For this review, take the finished solid that the model builds, in its own axes (mm). A direction names the side the tool comes from. Give positions to 0.01 mm unless a question says otherwise; leave off trailing zeros. Loops run counter-clockwise (first coordinate to the right, second up) from the corner with the lowest first, then second, coordinate; pieces in that order, holes last.
Autodesk Inventor part; units mm, degrees
ref_plane "Work Plane1" through (-110.3759, -8.6414, 0) normal (0, 1, 0) x (1, 0, 0)
ref_plane "YZ Plane" through (0, 0, 0) normal (1, 0, 0) x (0, 1, 0)
ref_plane "XZ Plane" through (0, 0, 0) normal (0, 1, 0) x (-1, 0, 0)
sketch "Sketch1" plane through (0, 0, 0) normal (0, 0, 1) x (1, 0, 0)
  line L0 (-110.3759, -8.6414) -> (42.0241, -8.6414)
  line L1 (42.0241, -8.6414) -> (42.0241, -59.4414)
  line L2 (42.0241, -59.4414) -> (-110.3759, -59.4414)
  circle A0 centre (-46.8759, -24.5164) radius 3.2512
  circle A1 centre (-46.8759, -43.5664) radius 3.2512
  line L3 (-13.5384, -25.7986) -> (-4.0134, -25.7986)
  line L4 (-4.0134, -25.7986) -> (0.7491, -34.0475)
  line L5 (0.7491, -34.0475) -> (-4.0134, -42.2964)
  line L6 (-4.0134, -42.2964) -> (-13.5384, -42.2964)
  line L7 (-13.5384, -42.2964) -> (-18.3009, -34.0475)
  line L8 (-18.3009, -34.0475) -> (-13.5384, -25.7986)
  circle A2 centre (-110.3759, -34.0414) radius 3.9751
  arc A3 (-110.3759, -8.6414) -> (-110.3759, -59.4414) centre (-110.3759, -34.0414) ccw
  point P0 (0, 0)
  point P1 (-8.7759, -34.0414)
  point P2 (-8.7759, -42.2964)
  dimension "d4" = 6.5024
  dimension "d5" = 6.5024
  dimension "d9" = 152.4
  dimension "d10" = 9.525
  dimension "d11" = 9.525
  dimension "d13" = 120
  dimension "d16" = 9.525
  dimension "d17" = 9.525
  dimension "d18" = 120
  dimension "d19" = 9.525
  dimension "d20" = 9.525
  dimension "d21" = 50.8
  dimension "d22" = 8.255
  dimension "d23" = 9.525
  dimension "d25" = 7.9502
  dimension "d27" = 9.525
  dimension "d37" = 19.05
  dimension "d38" = 50.8
  dimension "d39" = 25.4
  dimension "d40" = 63.5
  dimension "d51" = 101.6
extrude "Extrusion1" add sketch "Sketch1" along normal blind 10.16
ref_plane "Work Plane1" through (-110.3759, -8.6414, 0) normal (0, 1, 0) x (1, 0, 0)
sketch "Sketch3" plane through (-110.3759, -8.6414, 0) normal (0, 1, 0) x (1, 0, 0)
  line L0 (50.8, 1.8056) -> (50.8, -17.2484)
  line L1 (152.4, 0) -> (152.4, -10.16)
  circle A0 centre (76.2, -5.08) radius 3.175
  point P0 (110.3759, 0)
  point P1 (152.4, -5.08)
  dimension "d46" = 101.6
  dimension "d47" = 6.35
  dimension "d48" = 25.4
extrude "Extrusion2" cut sketch "Sketch3" against normal blind 50.8
sketch "Sketch4" plane through (42.0241, -59.4414, 0) normal (1, 0, 0) x (0, 0, -1)
  line L0 (-10.16, 0) -> (-10.16, 50.8)
  line L1 (0, 0) -> (0, 50.8)
  line L2 (-10.16, 50.8) -> (0, 50.8)
  line L3 (0, 50.8) -> (0, 0)
  line L4 (0, 0) -> (-10.16, 0)
  line L5 (-10.16, 0) -> (-10.16, 50.8)
  point P0 (0, 59.4414)
  point P1 (-10.16, 0)
extrude "Extrusion3" cut sketch "Sketch4" against normal blind 38.1
properties part number "new plates for arm"
Item 1: Tool access review of faces 1 (the flat face through (-54, -8.641, 5)), 2 (the flat face through (-1.665, -29.865, 5.009)): name each direction out of +Z, -Z, +X, -X, +Y, -Y from which nothing blocks a thin tool from reaching the whole face with its end or side.
Answer:
face 1: +Z, -Z, +X, -X, +Y
face 2: +Z, -Z
Item 2: Take a section at C-C on y = -19. Give the boundary of the cut face in (x, z) (3 decimals), and give its area (3 significant figures).
Answer:
outline: (-130.843, 0) - (3.924, 0) - (3.924, 10.16) - (-130.843, 10.16) - close; hole circle Ø6.35 at (-34.176, 5.08)
area: 1,340 mm2
Item 3: For L1, parallel to Y at x = -9, z = 7.25; L2, parallel to X at y = -42, z = 6.5; L3, parallel to X at y = -31, z = 5.08, list the stretches that pass through material, from the lowest coordinate up.
Answer:
L1: y = -59.44 to -42.3, -25.8 to -8.64
L2: x = -134.5 to -49.72, -44.03 to -37.02, -31.34 to -13.71, -3.84 to 3.92
L3: x = -135.59 to -112.94, -107.82 to -37.35, -31 to -16.54, -1.01 to 3.92
Item 4: Take a section at A-A on x = -11.5. Give the boundary of the cut face in (y, z), and give its area (3 significant figures).
Answer:
outline: (-59.44, 0) - (-42.3, 0) - (-42.3, 10.16) - (-59.44, 10.16) - close; (-25.8, 0) - (-8.64, 0) - (-8.64, 10.16) - (-25.8, 10.16) - close
area: 349 mm2
Item 5: Clearance check with flat-ended pins moving along their axes: pin 1 Ø5 at (y, z) = (-40, 1.5) entering from -X; pin 2 Ø8.5 at (x, y) = (-46.88, -24.52) entering from +Z. State where each tip first meets the part, or that it passes through.
Answer:
pin 1: stops at x = -135.54
pin 2: stops at z = 10.16
Item 6: Take a section at B-B on z = 5.08. Give the boundary of the cut face in (x, y), and give its area (3 significant figures).
Answer:
outline: (-110.38, -59.44) - (-37.35, -59.44) - (-37.35, -8.64) - (-110.38, -8.64) arc R25.4 ccw to start; (-31, -59.44) - (3.92, -59.44) - (3.92, -8.64) - (-31, -8.64) - close; hole circle Ø7.95 at (-110.38, -34.04); hole circle Ø6.5 at (-46.88, -43.57); hole circle Ø6.5 at (-46.88, -24.52); hole (-18.3, -34.05) - (-13.54, -42.3) - (-4.01, -42.3) - (0.75, -34.05) - (-4.01, -25.8) - (-13.54, -25.8) - close
area: 6,150 mm2
Item 7: The part is to be moulded in two halves that separate along X. For faces 3 (the flat face through (3.924, -34, 5)), 4 (the flat face through (-1.599, -38.114, 5.009)), 5 (the cylindrical face through (-135.77, -34.6, 5.01)), say which applies: released by +X, released by -X, zero draft, split by the parting line, or undercut.
Answer:
face 3: released by +X
face 4: undercut
face 5: released by -X
